Geometry: see drawing. Coordinates: mm, zero at the bounding-box minimum. A direction names the side the tool comes from. Coordinates: 2 decimals unless noted, no trailing zeros. Order: outer loops, then holes, each group sorted by start corner. A loop starts at its lowest first (then second) coordinate and runs counter-clockwise, first axis right, second up. Notation, with made-up numbers: (89, -18.75) -> (144, -18.75) arc R23 ccw to (144, -3.75) -> close; hole circle Ø2 at (4, 87). An arc over 180 degrees is marked (long way). One line per item, written item: value. Start each with the question number.
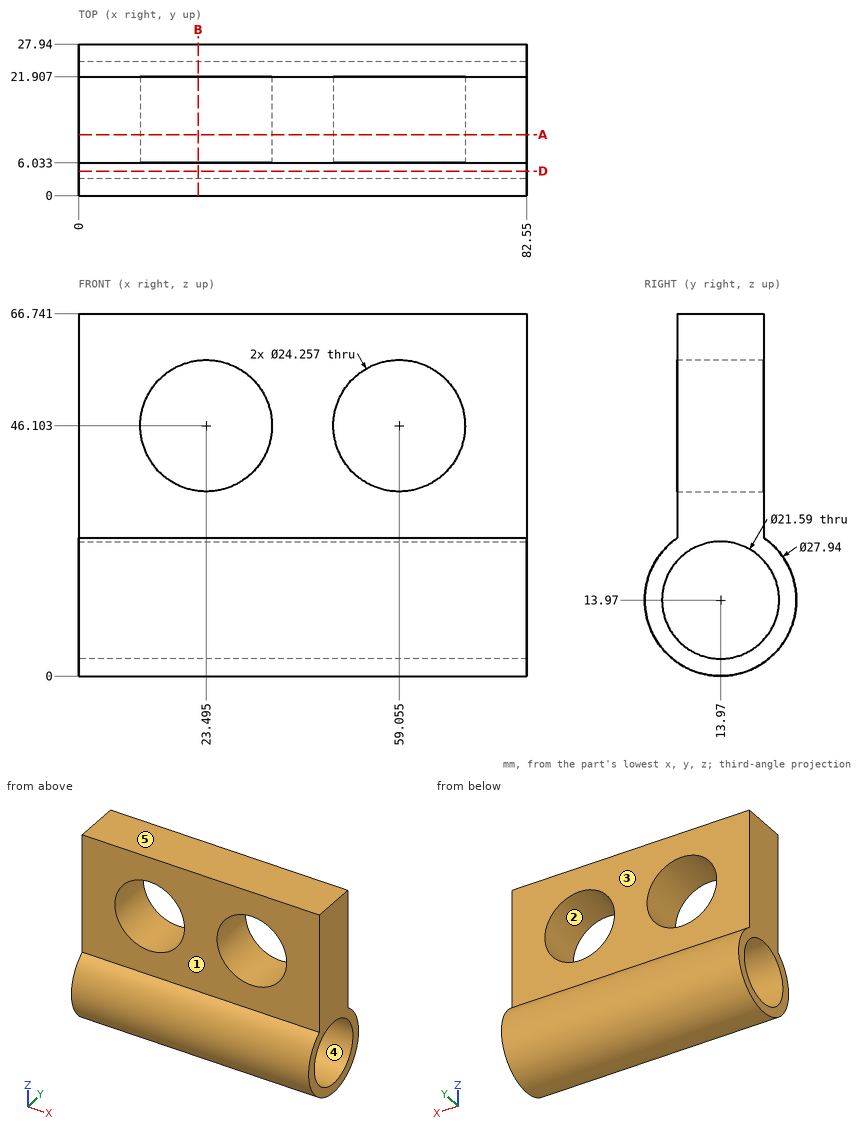
1) Ray query, line 1 along Z through (x, y) = (19, 11.75) (1 decimal); line 2 along X through (y, z) = (16.25, 50.5); line 3 along X through (y, z) = (17.5, 43). Return the intervals inside material, ascending. Write a range as from..to.
2) Section query A-A, the plane y = 11.25. State how many separate pieces and enclosed holes the cut face has, plus the area to 3 significant figures.
3) Section query D-D, the plane y = 4.5. Return the cut outline in (x, z), plus the area to 3 significant figures.
4) Pin query (flat end, axial travel): pin 1 Ø1 at (x, z) = (64, 13) entering from -Y; pin 2 Ø12 at (x, y) = (23.5, 22) entering from +Z; pin 3 Ø5 at (x, z) = (14, 23.5) entering from +Y; pin 4 Ø4 at (x, y) = (29.5, 24) entering from +Z. Return the tip coordinate at first contact, or that it passes through.
5) Access query for the marked faces 1 and 2. Directions: +Z, -Z, +X, -X, +Y, -Y. A direction counts if a zero-diameter tool reaches every point of the face in a straight line with its end or side. Return the directions, or none.
6) Section query B-B, the plane x = 22. Return the cut outline in (y, z) (1 decimal).
7) Mould query, pull axis Z, two halves, no side actions, for the marked faces 3, 4 and 5. Classes: +Z half, -Z half, draft (parallel to the pull), parting line (faces both ways), or undercut.
Entries:
1. line 1: z = 0.2..3.4, 24.5..34.8, 57.4..66.7
1. line 2: x = 0..12.19, 34.8..47.75, 70.36..82.55
1. line 3: x = 0..11.77, 35.22..47.33, 70.78..82.55
2. separate pieces: 2
2. enclosed holes: 2
2. area: 2,840 mm2
3. outline: (0, 3.7) -> (82.55, 3.7) -> (82.55, 8.79) -> (0, 8.79) -> close; (0, 19.15) -> (82.55, 19.15) -> (82.55, 24.24) -> (0, 24.24) -> close
3. area: 840 mm2
4. pin 1: stops at y = 0.01
4. pin 2: stops at z = 66.74
4. pin 3: stops at y = 26.04
4. pin 4: stops at z = 25.4
5. face 1: +Z, +X, -X, -Y
5. face 2: +Y, -Y
6. outline: (6, 25.5) arc R14 ccw (long way) to (21.9, 25.5) -> (21.9, 34.1) -> (6, 34.1) -> close; (6, 58.1) -> (21.9, 58.1) -> (21.9, 66.7) -> (6, 66.7) -> close; hole circle Ø21.6 at (14, 14)
7. face 3: draft
7. face 4: undercut
7. face 5: +Z half
